```python
from build123d import *

# Parameters (mm, degrees)
SKETCH1_W           = 40
SKETCH1_H           = 30
BOSS_EXTRUDE1_DEPTH = 50
SKETCH3_W           = 33
SKETCH3_H           = 23
CUT_EXTRUDE1_DEPTH  = 51
SKETCH4_R           = 1.25
CUT_EXTRUDE2_DEPTH  = 10


with BuildPart() as part:
    # Sketch1 → Boss-Extrude1 (new body)
    with BuildSketch(Plane.XY):
        with Locations((20, 15)):
            Rectangle(SKETCH1_W, SKETCH1_H)
    extrude(amount=BOSS_EXTRUDE1_DEPTH)

    # Sketch3 → Cut-Extrude1 (cut, through all)
    with BuildSketch(Plane.XY.offset(50)):
        with Locations((20, 15)):
            Rectangle(SKETCH3_W, SKETCH3_H)
    extrude(amount=-CUT_EXTRUDE1_DEPTH, mode=Mode.SUBTRACT)

    # Sketch4 → Cut-Extrude2 (cut)
    with BuildSketch(Plane.XY.offset(50)):
        with Locations((38, 28)):
            Circle(SKETCH4_R)
        with Locations((2, 28)):
            Circle(SKETCH4_R)
        with Locations((2, 2)):
            Circle(SKETCH4_R)
        with Locations((38, 2)):
            Circle(SKETCH4_R)
    extrude(amount=-CUT_EXTRUDE2_DEPTH, mode=Mode.SUBTRACT)


solid = part.part
```
The listing builds one solid part. Answer for the finished solid, in the listing's coordinates (mm). A direction names the side the tool comes from. Give positions to 0.01 mm unless a question says otherwise; leave off trailing zeros. Order: outer loops, then holes, each group sorted by start corner. A loop starts at its lowest first (then second) coordinate and runs counter-clockwise, first axis right, second up.
Item 1: The part is cut by section A-A, the plane x = 5. Give the vertices of the cut face in (y, z), and give its area (3 significant figures).
From the geometry:
outline: (0, 0) - (3.5, 0) - (3.5, 50) - (0, 50) - close; (26.5, 0) - (30, 0) - (30, 50) - (26.5, 50) - close
area: 350 mm2
Item 2: Given pin 1 Ø2 at (x, y) = (2, 2) entering from +Z, flat-ended and moving along its own axis, determine where the tip first touches the part or whether it passes through.
From the geometry:
pin 1: stops at z = 40
Item 3: Find the intervals of material crossed by probe 1 along Y at (x, z) = (2, 46); probe 2 along X at (y, z) = (24.5, 30); probe 3 along Y at (x, z) = (21, 4), in increasing order.
From the geometry:
probe 1: y = 0 to 0.75, 3.25 to 26.75, 29.25 to 30
probe 2: x = 0 to 3.5, 36.5 to 40
probe 3: y = 0 to 3.5, 26.5 to 30
Item 4: For a pull along X with two mould halves and no side action, classify faces 1 (the face through (3.19, 28.38, 45.07)), 2 (the face through (20, 0, 25)), 3 (the face through (0, 15, 25)) as pulls with the +X half, pulls with the -X half, needs draft (parallel to the pull), parting line crosses it, or undercut.
From the geometry:
face 1: undercut
face 2: needs draft
face 3: pulls with the -X half
Item 5: The part is cut by section B-B, the plane y = 12.25. Give the vertices of the cut face in (x, z), and give its area (3 significant figures).
From the geometry:
outline: (0, 0) - (3.5, 0) - (3.5, 50) - (0, 50) - close; (36.5, 0) - (40, 0) - (40, 50) - (36.5, 50) - close
area: 350 mm2
Item 6: Which of the six approach directions +Z, -Z, +X, -X, +Y, -Y give full straight-line access (tool end or side, diameter ignored) to faces 4 (the face through (20, 26.5, 25)), 5 (the face through (36.75, 28.05, 45.07)), 6 (the face through (40, 15, 25))?
From the geometry:
face 4: +Z, -Z
face 5: +Z
face 6: +Z, -Z, +X, +Y, -Y
Item 7: The part is cut by section C-C, the plane z = 20. Give the vertices of the cut face in (x, y), and give its area (3 significant figures).
From the geometry:
outline: (0, 0) - (40, 0) - (40, 30) - (0, 30) - close; hole (3.5, 3.5) - (36.5, 3.5) - (36.5, 26.5) - (3.5, 26.5) - close
area: 441 mm2
Item 8: The part is cut by section D-D, the plane y = 28. Give the vertices of the cut face in (x, z), and give its area (3 significant figures).
From the geometry:
outline: (0, 0) - (40, 0) - (40, 50) - (39.25, 50) - (39.25, 40) - (36.75, 40) - (36.75, 50) - (3.25, 50) - (3.25, 40) - (0.75, 40) - (0.75, 50) - (0, 50) - close
area: 1,950 mm2
